from build123d import *

# Parameters (mm, degrees)
SKETCH2_R           = 13
SKETCH2_R_2         = 3
BOSS_EXTRUDE1_DEPTH = 11


with BuildPart() as part:
    # Sketch2 → Boss-Extrude1 (new body)
    with BuildSketch(Plane.XY):
        with BuildLine():
            Line((0, 0), (75, 0))
            Line((75, 0), (75, 120))
            ThreePointArc((75, 120), (72.071067812, 127.071067812), (65, 130))
            Line((65, 130), (10, 130))
            ThreePointArc((10, 130), (2.928932188, 127.071067812), (0, 120))
            Line((0, 120), (0, 0))
        make_face()
        with Locations((37.5, 90)):
            Circle(SKETCH2_R, mode=Mode.SUBTRACT)
        with Locations((61.291446946, 103.286442421)):
            Circle(SKETCH2_R_2, mode=Mode.SUBTRACT)
        with Locations((14.097879865, 103.960776238)):
            Circle(SKETCH2_R_2, mode=Mode.SUBTRACT)
        with Locations((37.110673189, 62.752781341)):
            Circle(SKETCH2_R_2, mode=Mode.SUBTRACT)
    extrude(amount=BOSS_EXTRUDE1_DEPTH)


solid = part.part
Check sheet for the modelled part. Datum: model origin and axes. Units: mm. Give positions to 0.01 mm unless a question says otherwise; leave off trailing zeros. Write each loop counter-clockwise with the first axis right and the second up, starting at its lowest first coordinate (ties: lowest second). Pieces come first, ordered by that corner, then holes. Notation, with made-up numbers: (32, 67) -> (82, 67) arc R28 cw to (82, 91) -> close; hole circle Ø8 at (-13, 74). An arc over 180 degrees is marked (long way). Use one line per item in the form item = value. Start each with the question number.
1. Go/stop test with a flat-tipped pin: P1, Ø9.5, axis at x = 61.29, y = 103.29, coming from the -Z side. Record where the tip stops, or that it passes through.
2. Mould release check, pull along X, two halves, no side actions. Record for faces 1 (the cylindrical face through (11.717, 102.135, 5.423)), 2 (the cylindrical face through (72.15, 126.99, 5.42)), 3 (the flat face through (37, 66, 0)): pulls with the +X half, pulls with the -X half, needs draft (parallel to the pull), parting line crosses it, or undercut.
3. Thickness scan on line 1 along Y through (x, z) = (13, 10); line 2 along Y through (x, z) = (45.5, 6); line 3 along X through (y, z) = (81, 6.25). Record the ranges inside material, lowest first. Write a range as from..to.
4. Section check A-A (x = 32.5). Record the cut outline in (y, z), and give its area (3 significant figures).
5. Section check C-C (z = 4.5). Record the cut outline in (x, y).
6. Section check B-B (y = 90). Record the cut outline in (x, z), and give its area (3 significant figures).
Conclusion:
q1.P1 = 0
q2.face_1 = undercut
q2.face_2 = pulls with the +X half
q2.face_3 = needs draft
q3.line_1 = 0..101.17, 106.75..130
q3.line_2 = 0..79.75, 100.25..130
q3.line_3 = 0..28.12, 46.88..75
q4.outline = (0, 0) -> (78, 0) -> (78, 11) -> (0, 11) -> close; (102, 0) -> (130, 0) -> (130, 11) -> (102, 11) -> close
q4.area = 1,170 mm²
q5.outline = (0, 0) -> (75, 0) -> (75, 120) arc R10 ccw to (65, 130) -> (10, 130) arc R10 ccw to (0, 120) -> close; hole circle Ø6 at (14.1, 103.96); hole circle Ø26 at (37.5, 90); hole circle Ø6 at (37.11, 62.75); hole circle Ø6 at (61.29, 103.29)
q6.outline = (0, 0) -> (24.5, 0) -> (24.5, 11) -> (0, 11) -> close; (50.5, 0) -> (75, 0) -> (75, 11) -> (50.5, 11) -> close
q6.area = 539 mm²
